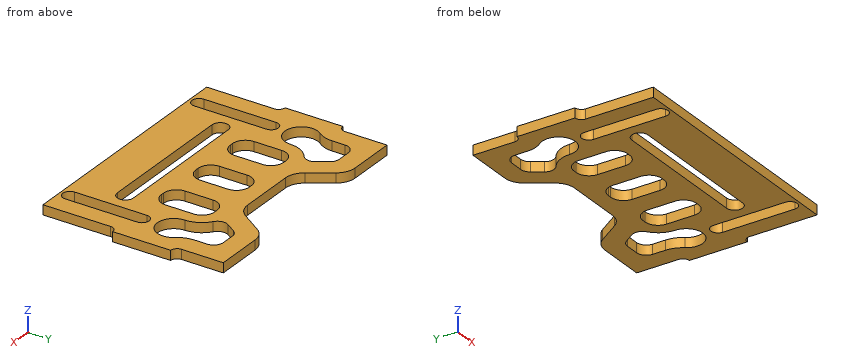
from build123d import *

# Parameters (mm, degrees)
F1_DEPTH = 1.5


# Not quite as in the source:
# - ends of sketch curves that miss each other by under 0.0002 mm in the source are joined


with BuildPart() as f1:
    # F0 (on Top) → F1 (new body)
    with BuildSketch(Plane.XY):
        with BuildLine():
            ThreePointArc((20, 6.5), (19.2928932188, 6.7928932188), (19, 7.5))
            Line((19, 7.5), (19, 14))
            Line((19, 14), (11.605551, 14))
            ThreePointArc((11.605551, 14), (10.1899773457, 13.6450238617), (9.1094002708, 12.6641008194))
            Line((9.1094002708, 12.6641008194), (6.890599, 9.3359))
            ThreePointArc((6.890599, 9.3359), (5.8100220211, 8.3549763346), (4.394448, 8))
            Line((4.394448, 8), (-4.394449, 8))
            ThreePointArc((-4.394449, 8), (-5.8100230211, 8.3549763346), (-6.8906001907, 9.3358998729))
            Line((-6.8906001907, 9.3358998729), (-9.109401, 12.664101))
            ThreePointArc((-9.109401, 12.664101), (-10.1899783457, 13.6450238617), (-11.605552, 14))
            Line((-11.605552, 14), (-19, 14))
            Line((-19, 14), (-19, 7.5))
            ThreePointArc((-19, 7.5), (-19.2928932188, 6.7928932188), (-20, 6.5))
            Line((-20, 6.5), (-20, -2.5))
            ThreePointArc((-20, -2.5), (-19.2928932188, -2.7928932188), (-19, -3.5))
            Line((-19, -3.5), (-19, -14))
            Line((-19, -14), (19, -14))
            Line((19, -14), (19, -3.5))
            ThreePointArc((19, -3.5), (19.2928932188, -2.7928932188), (20, -2.5))
            Line((20, -2.5), (20, 6.5))
        make_face()
        with BuildLine():
            ThreePointArc((-13.9, -12.498995), (-15, -13.598995), (-16.1, -12.498995))
            Line((-16.1, -12.498995), (-16.1, -1.300086))
            ThreePointArc((-16.1, -1.300086), (-15, -0.200086), (-13.9, -1.300086))
            Line((-13.9, -1.300086), (-13.9, -12.498995))
        make_face(mode=Mode.SUBTRACT)
        with BuildLine():
            ThreePointArc((-11, -7.808873), (-12.25, -6.558873), (-11, -5.308873))
            Line((-11, -5.308873), (11, -5.308873))
            ThreePointArc((11, -5.308873), (12.25, -6.558873), (11, -7.808873))
            Line((11, -7.808873), (-11, -7.808873))
        make_face(mode=Mode.SUBTRACT)
        with BuildLine():
            ThreePointArc((16.1, -12.498995), (15, -13.598995), (13.9, -12.498995))
            Line((13.9, -12.498995), (13.9, -1.300086))
            ThreePointArc((13.9, -1.300086), (15, -0.200086), (16.1, -1.300086))
            Line((16.1, -1.300086), (16.1, -12.498995))
        make_face(mode=Mode.SUBTRACT)
        with BuildLine():
            ThreePointArc((-12.25, 3.5), (-15.6295091101, 1.0805038434), (-16.8308317088, 5.0594317757))
            ThreePointArc((-16.8308317088, 5.0594317757), (-16.2134004171, 6.2109446874), (-16, 7.5))
            Line((-16, 7.5), (-16, 9.5))
            ThreePointArc((-16, 9.5), (-15.5606601718, 10.5606601718), (-14.5, 11))
            Line((-14.5, 11), (-12.408327, 11))
            ThreePointArc((-12.408327, 11), (-11.7005404785, 10.8225120945), (-11.16025202, 10.3320509866))
            Line((-11.16025202, 10.3320509866), (-10.161512, 8.83394))
            ThreePointArc((-10.161512, 8.83394), (-9.935298233, 7.7253531463), (-10.5478817855, 6.7741016944))
            ThreePointArc((-10.5478817855, 6.7741016944), (-11.7990510276, 5.3450573983), (-12.25, 3.5))
        make_face(mode=Mode.SUBTRACT)
        with BuildLine():
            Line((-5.75, 3.5), (-5.75, -0.808873))
            ThreePointArc((-5.75, -0.808873), (-6.3357864376, -2.2230865624), (-7.75, -2.808873))
            Line((-7.75, -2.808873), (-8.25, -2.808873))
            ThreePointArc((-8.25, -2.808873), (-9.6642135624, -2.2230865624), (-10.25, -0.808873))
            Line((-10.25, -0.808873), (-10.25, 3.5))
            ThreePointArc((-10.25, 3.5), (-9.6642135624, 4.9142135624), (-8.25, 5.5))
            Line((-8.25, 5.5), (-7.75, 5.5))
            ThreePointArc((-7.75, 5.5), (-6.3357864376, 4.9142135624), (-5.75, 3.5))
        make_face(mode=Mode.SUBTRACT)
        with BuildLine():
            Line((2.25, 3.5), (2.25, -0.808873))
            ThreePointArc((2.25, -0.808873), (1.6642135624, -2.2230865624), (0.25, -2.808873))
            Line((0.25, -2.808873), (-0.25, -2.808873))
            ThreePointArc((-0.25, -2.808873), (-1.6642135624, -2.2230865624), (-2.25, -0.808873))
            Line((-2.25, -0.808873), (-2.25, 3.5))
            ThreePointArc((-2.25, 3.5), (-1.6642135624, 4.9142135624), (-0.25, 5.5))
            Line((-0.25, 5.5), (0.25, 5.5))
            ThreePointArc((0.25, 5.5), (1.6642135624, 4.9142135624), (2.25, 3.5))
        make_face(mode=Mode.SUBTRACT)
        with BuildLine():
            Line((10.25, 3.5), (10.25, -0.808873))
            ThreePointArc((10.25, -0.808873), (9.6642135624, -2.2230865624), (8.25, -2.808873))
            Line((8.25, -2.808873), (7.75, -2.808873))
            ThreePointArc((7.75, -2.808873), (6.3357864376, -2.2230865624), (5.75, -0.808873))
            Line((5.75, -0.808873), (5.75, 3.5))
            ThreePointArc((5.75, 3.5), (6.3357864376, 4.9142135624), (7.75, 5.5))
            Line((7.75, 5.5), (8.25, 5.5))
            ThreePointArc((8.25, 5.5), (9.6642135624, 4.9142135624), (10.25, 3.5))
        make_face(mode=Mode.SUBTRACT)
        with BuildLine():
            ThreePointArc((16.8308313365, 5.0594322592), (15.6295093989, 1.0805039417), (12.25, 3.5))
            ThreePointArc((12.25, 3.5), (11.7990508389, 5.3450577615), (10.5478809284, 6.774101898))
            ThreePointArc((10.5478809284, 6.774101898), (9.9352982087, 7.7253532759), (10.1615112508, 8.8339398328))
            Line((10.1615112508, 8.8339398328), (11.160251, 10.332051))
            ThreePointArc((11.160251, 10.332051), (11.700540234, 10.8225119636), (12.408327, 11))
            Line((12.408327, 11), (14.5, 11))
            ThreePointArc((14.5, 11), (15.5606601718, 10.5606601718), (16, 9.5))
            Line((16, 9.5), (16, 7.5))
            ThreePointArc((16, 7.5), (16.2134003188, 6.2109449762), (16.8308313365, 5.0594322592))
        make_face(mode=Mode.SUBTRACT)
    extrude(amount=F1_DEPTH)


solid = f1.part
Geometry: final body of the model. Coordinates: model frame, mm. Give positions to 0.01 mm unless a question says otherwise; leave off trailing zeros. Loops run counter-clockwise (first coordinate to the right, second up) from the corner with the lowest first, then second, coordinate; pieces in that order, holes last. Notation, with made-up numbers: (67.25, 66) -> (80.25, 66) arc R20 cw to (80.25, 70) -> close; hole circle Ø5 at (-20.5, -7.75). An arc over 180 degrees is marked (long way). Put each result on its own line as item: value.
1. Pin query (flat end, axial travel): P1, Ø0.8, axis at y = 9.5, z = 1, coming from the +X side; P2, Ø0.8, axis at x = -5, z = 0.5, coming from the +Y side. Return the tip coordinate at first contact, or that it passes through.
Taken from the geometry:
P1: stops at x = 19
P2: stops at y = 8.17
2. Cut plane D-D (x = 1). Return the cut outline in (y, z), plus the area to 3 significant figures.
Taken from the geometry:
outline: (-14, 0) -> (-7.81, 0) -> (-7.81, 1.5) -> (-14, 1.5) -> close; (-5.31, 0) -> (-2.66, 0) -> (-2.66, 1.5) -> (-5.31, 1.5) -> close; (5.35, 0) -> (8, 0) -> (8, 1.5) -> (5.35, 1.5) -> close
area: 17.2 mm2
3. Cut plane B-B (z = 0.25). Count the separate pieces of the cut face and the enclosed holes in it, plus the area to 3 significant figures.
Taken from the geometry:
separate pieces: 1
enclosed holes: 8
area: 669 mm2
4. Ray query, line 1 along X through (y, z) = (3.5, 1.2); line 2 along X through (y, z) = (-8.5, 0.3); line 3 along X through (y, z) = (-6.5, 1.1). Return the intervals inside material, ascending. Write a range as [from, to].
Taken from the geometry:
line 1: x = [-20, -17.36], [-12.25, -10.25], [-5.75, -2.25], [2.25, 5.75], [10.25, 12.25], [17.36, 20]
line 2: x = [-19, -16.1], [-13.9, 13.9], [16.1, 19]
line 3: x = [-19, -16.1], [-13.9, -12.25], [12.25, 13.9], [16.1, 19]
5. Cut plane A-A (x = -15). Return the cut outline in (y, z).
Taken from the geometry:
outline: (-14, 0) -> (-13.6, 0) -> (-13.6, 1.5) -> (-14, 1.5) -> close; (-0.2, 0) -> (0.95, 0) -> (0.95, 1.5) -> (-0.2, 1.5) -> close; (10.91, 0) -> (14, 0) -> (14, 1.5) -> (10.91, 1.5) -> close
6. Cut plane C-C (y = -6). Return the cut outline in (x, z), plus the area to 3 significant figures.
Taken from the geometry:
outline: (-19, 0) -> (-16.1, 0) -> (-16.1, 1.5) -> (-19, 1.5) -> close; (-13.9, 0) -> (-12.12, 0) -> (-12.12, 1.5) -> (-13.9, 1.5) -> close; (12.12, 0) -> (13.9, 0) -> (13.9, 1.5) -> (12.12, 1.5) -> close; (16.1, 0) -> (19, 0) -> (19, 1.5) -> (16.1, 1.5) -> close
area: 14.0 mm2
